Can you work these out from the model? Positions are in its coordinate system, mm. Face numbers are marked on the shaded views. A direction names the side the tool comes from. Give positions to 0.01 mm unless a question says otherwise; leave off trailing zeros. Write each loop counter-clockwise with the first axis right and the second up, starting at its lowest first coordinate (ties: lowest second). Pieces come first, ordered by that corner, then holes. Notation, with made-up numbers: (53.25, 54.5) -> (97.25, 54.5) arc R26 ccw to (97.25, 78.5) -> close; hole circle Ø10 at (56.5, 37). An arc over 180 degrees is marked (long way). One line per item, written item: value.
from build123d import *

# Parameters (mm, degrees)
F0_R     = 22
F2_R     = 25
F4_R     = 12.25
F5_DEPTH = 25.001
F4_R_2   = 22
F4_R_3   = 15.25
F6_DEPTH = 10
F7_R     = 3


with BuildPart() as f3:
    # F0 (on Top) → F3 section 0
    with BuildSketch(Plane.XY):
        Circle(F0_R)
    # F2 (on offset) → F3 section 1
    with BuildSketch(Plane.XY.offset(25)):
        Circle(F2_R)
    loft()

    # F4 (on offset) → F5 (cut, through all)
    with BuildSketch(Plane.XY.offset(25)):
        Circle(F4_R)
    extrude(amount=-F5_DEPTH, mode=Mode.SUBTRACT)

    # F4 (on offset) → F6 (cut)
    with BuildSketch(Plane.XY.offset(25)):
        Circle(F4_R_2)
        Circle(F4_R_3, mode=Mode.SUBTRACT)
    extrude(amount=-F6_DEPTH, mode=Mode.SUBTRACT)

    # F7
    f7_edges = [f3.edges().sort_by_distance(p)[0] for p in [
        (-22, 0, 15),
        (-15.25, 0, 15),
    ]]
    fillet(f7_edges, radius=F7_R)


solid = f3.part
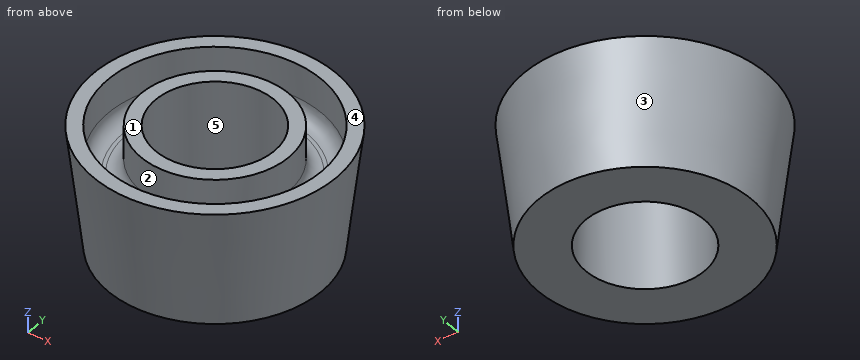
1) If we section it at C-C (z = 4.5): Write out the boundary of the cut face in (x, y), and give its area (3 significant figures).
Answer list:
outline: circle Ø45.08 at (0, 0); hole circle Ø24.5 at (0, 0)
area: 1,120 mm^2
2) If we section it at D-D (z = 8): Write out the boundary of the cut face in (x, y).
Answer list:
outline: circle Ø45.92 at (0, 0); hole circle Ø24.5 at (0, 0)
3) We'd pull the mould along Y, two halves only. Please class the marked faces 3, 4 and 5: released by +Y, released by -Y, zero draft, split by the parting line, or undercut.
Answer list:
face 3: split by the parting line
face 4: zero draft
face 5: undercut
4) Will these pins go through, and if not, where does the flat tip stop? pin 1 (4 mm diameter, centred on x = -2.5, z = 2.5, fed in from -Y); pin 2 (2 mm diameter, centred on y = -8, z = 18.5, fed in from +X); pin 3 (10 mm diameter, centred on x = 18.5, z = 19, fed in from -Y).
Answer list:
pin 1: stops at y = -22.46
pin 2: stops at x = 23.21
pin 3: stops at y = -20.26
5) If we section it at B-B (z = 21.5): Write out the boundary of the cut face in (x, y).
Answer list:
outline: circle Ø49.16 at (0, 0); circle Ø30.5 at (0, 0); hole circle Ø44 at (0, 0); hole circle Ø24.5 at (0, 0)
6) If we section it at A-A (x = 0): Write out the boundary of the cut face in (y, z), and give its area (3 significant figures).
Answer list:
outline: (-25, 25) -> (-22, 0) -> (-12.25, 0) -> (-12.25, 25) -> (-15.25, 25) -> (-15.25, 18) arc R3 cw to (-18.25, 15) -> (-19, 15) arc R3 cw to (-22, 18) -> (-22, 25) -> close; (12.25, 0) -> (22, 0) -> (25, 25) -> (22, 25) -> (22, 18) arc R3 cw to (19, 15) -> (18.25, 15) arc R3 cw to (15.25, 18) -> (15.25, 25) -> (12.25, 25) -> close
area: 435 mm^2
7) I need wall thicknesses on L1, parallel to X at y = 9.5, z = 23; L2, parallel to Y at x = -6, z = 15.5; L3, parallel to X at y = -13.5, z = 21.25. Which ranges of each line are inside material? Lowest first, please.
Answer list:
L1: x = -22.86 to -19.84, -11.93 to -7.73, 7.73 to 11.93, 19.84 to 22.86
L2: y = -23.09 to -19.77, -15.47 to -10.68, 10.68 to 15.47, 19.77 to 23.09
L3: x = -20.5 to -17.37, -7.09 to 7.09, 17.37 to 20.5
8) For the marked faces 1 and 2, which set-ups out of +Z, -Z, +X, -X, +Y, -Y let a thin tool reach every point of the face, with its end or its side?
Answer list:
face 1: +Z, +X, -X, +Y, -Y
face 2: +Z
